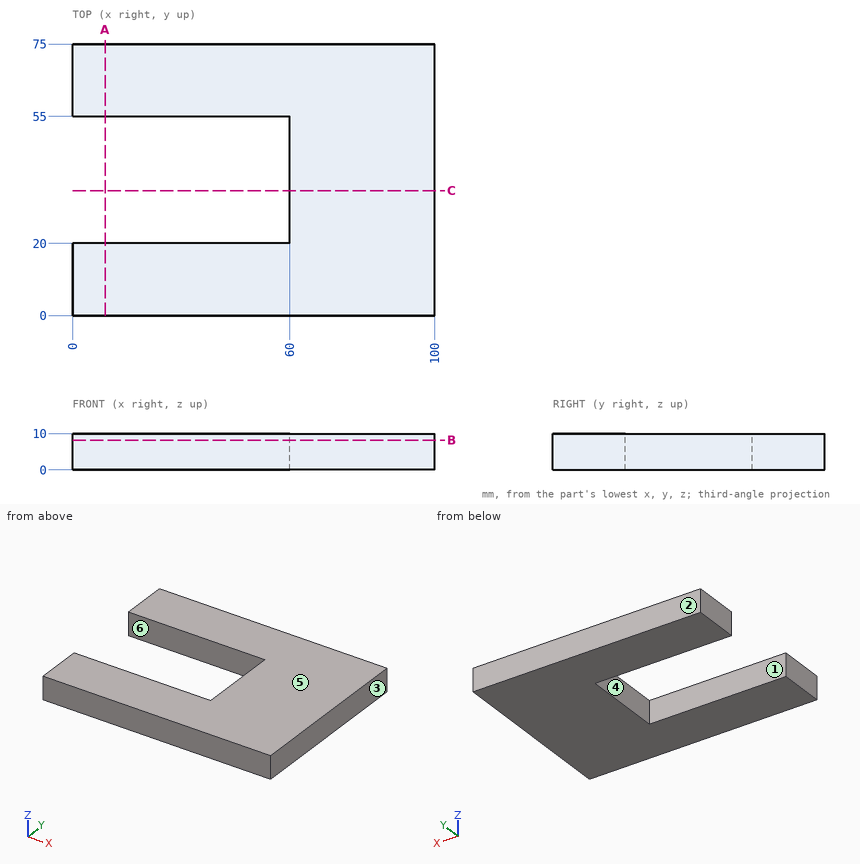
Source: three-view drawing plus pictorial views. Frame: mm from the lowest corner of the part. A direction names the side the tool comes from. Round coordinates to 2 decimals unless told otherwise and drop trailing zeros. Loops run counter-clockwise (first coordinate to the right, second up) from the corner with the lowest first, then second, coordinate; pieces in that order, holes last.
1. Contact query for a flat-ended pin moving along its axis: pin 1 (5 mm diameter, centred on y = 33.5, z = 3, fed in from -X). Output: stop coordinate, or through.
2. Section query B-B on z = 8.25. Output: boundary loops of the cut face in (x, y).
3. Mould query, pull axis Y, two halves, no side actions, for the marked faces 1, 2, 3 and 4. Classes: released by +Y, released by -Y, zero draft, split by the parting line, or undercut.
4. Access query for the marked faces 5 and 6. Directions: +Z, -Z, +X, -X, +Y, -Y. A direction counts if a zero-diameter tool reaches every point of the face in a straight line with its end or side. Return the directions, or none.
5. Ray query, L1, parallel to Y at x = 49, z = 5; L2, parallel to X at y = 21, z = 3.25. Return the intervals inside material, ascending.
6. Section query A-A on x = 9. Output: boundary loops of the cut face in (y, z), and give its area (3 significant figures).
7. Section query C-C on y = 34.5. Output: boundary loops of the cut face in (x, z).
Answers below:
1. pin 1: stops at x = 60
2. outline: (0, 0) - (100, 0) - (100, 75) - (0, 75) - (0, 55) - (60, 55) - (60, 20) - (0, 20) - close
3. face 1: undercut
3. face 2: released by +Y
3. face 3: zero draft
3. face 4: undercut
4. face 5: +Z, +X, -X, +Y, -Y
4. face 6: +Z, -Z, -X
5. L1: y = 0 to 20, 55 to 75
5. L2: x = 60 to 100
6. outline: (0, 0) - (20, 0) - (20, 10) - (0, 10) - close; (55, 0) - (75, 0) - (75, 10) - (55, 10) - close
6. area: 400 mm2
7. outline: (60, 0) - (100, 0) - (100, 10) - (60, 10) - close
